Read the model definition and answer for the solid it produces. Units are mm, in the model's axes. Face numbers are marked on the shaded views. A direction names the side the tool comes from. Round coordinates to 2 decimals unless told otherwise and drop trailing zeros. Loops run counter-clockwise (first coordinate to the right, second up) from the corner with the lowest first, then second, coordinate; pieces in that order, holes last. Notation, with made-up numbers: M 16.5,-25.75 L 38.5,-25.75 A21 cw 38.5,1.25 Z; hole C -13,62.5 d4. An arc over 180 degrees is marked long. Write each question's results on one line, items separated by ' | '.
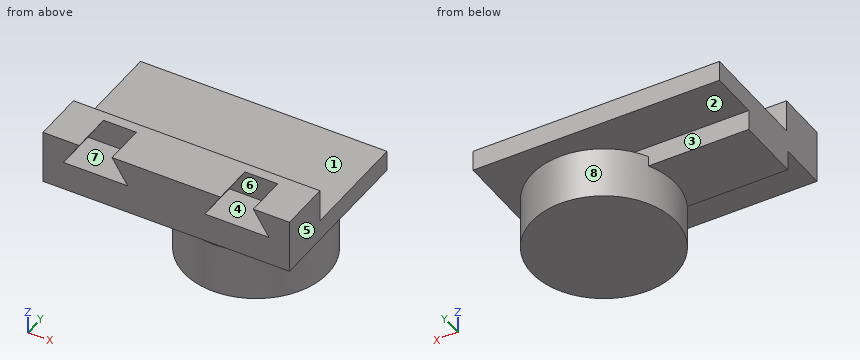
```python
from build123d import *

# Parameters (mm, degrees)
F0_W      = 38.1
F0_H      = 25.4
F1_DEPTH  = 3.175
F3_DEPTH  = 6.35
F4_W      = 38.1
F4_H      = 1.5875
F5_DEPTH  = 5.08
F6_R      = 11.1125
F7_DEPTH  = 9.525
F8_R      = 11.43
F8_R_2    = 7.62
F9_DEPTH  = 1.5875
F10_W     = 19.05
F10_H     = 10.16
F11_DEPTH = 3.175


with BuildPart() as f1:
    # F0 (on Top) → F1 (new body)
    with BuildSketch(Plane.XY):
        with Locations((-19.05, 12.7)):
            Rectangle(F0_W, F0_H)
    extrude(amount=F1_DEPTH)

    # F2 (on face) → F3 (join)
    with BuildSketch(Plane.XZ):
        Polygon((-38.1, 8.255), (-38.1, 3.175), (0, 3.175), (0, 8.255), (-5.588, 8.255), (-3.175, 4.445), (-13.081, 4.445), (-10.668, 8.255), (-27.432, 8.255), (-25.019, 4.445), (-34.925, 4.445), (-32.512, 8.255), align=None)
    extrude(amount=-F3_DEPTH)

    # F4 (on face) → F5 (join, through all)
    with BuildSketch(Plane.XY.offset(3.175)):
        with Locations((-19.05, 7.14375)):
            Rectangle(F4_W, F4_H)
    extrude(amount=F5_DEPTH)

    # F6 (on face) → F7 (join)
    with BuildSketch(Plane(origin=(0, 0, 0), x_dir=(1, 0, 0), z_dir=(0, 0, -1))):
        with Locations((-12.7, -12.7)):
            Circle(F6_R)
    extrude(amount=F7_DEPTH)

    # F8 (on face) → F9 (cut)
    with BuildSketch(Plane(origin=(0, 0, 0), x_dir=(1, 0, 0), z_dir=(0, 0, -1))):
        with Locations((-12.7, -12.7)):
            Circle(F8_R)
        with Locations((-12.7, -12.7)):
            Circle(F8_R_2, mode=Mode.SUBTRACT)
    extrude(amount=F9_DEPTH, mode=Mode.SUBTRACT)

    # F10 (on face) → F11 (join)
    with BuildSketch(Plane(origin=(0, 0, 0), x_dir=(1, 0, 0), z_dir=(0, 0, -1))):
        with Locations((-28.575, -12.7)):
            Rectangle(F10_W, F10_H)
    extrude(amount=F11_DEPTH)


solid = f1.part
```
1. Find section C-C, the plane y = 12.7. Give the vertices of the cut face in (x, z) (1 decimal), then the cut area to 3 significant figures.
Completed:
outline: M -38.1,-3.2 L -23.8,-3.2 L -23.8,-9.5 L -1.6,-9.5 L -1.6,-1.6 L -5.1,-1.6 L -5.1,0 L 0,0 L 0,3.2 L -38.1,3.2 Z | area: 372 mm2
2. Find section D-D, the plane z = -5.5. Give the vertices of the cut face in (x, y) (1 decimal), then the cut area to 3 significant figures.
Completed:
outline: C -12.7,12.7 d22.2 | area: 388 mm2
3. Find section A-A, the plane y = 22.5. Give the vertices of the cut face in (x, z) (1 decimal), then the cut area to 3 significant figures.
Completed:
outline: M -38.1,0 L 0,0 L 0,3.2 L -38.1,3.2 Z; M -17.9,-9.5 L -7.5,-9.5 L -7.5,-1.6 L -17.9,-1.6 Z | area: 204 mm2
4. Given P1, Ø6.5, axis at x = -16.5, y = 18, coming from the +Z side (3 decimals); P2, Ø1.9, axis at x = -9, z = 7, coming from the -Y side; P3, Ø1, axis at y = 17.5, z = -1, coming from the +X side, each flat-ended and moving along its own axis, determine where each tip first touches the part or whether it passes through.
Completed:
P1: stops at z = 3.175 | P2: stops at y = 6.35 | P3: stops at x = -6.41
5. Determine the mould class of the marked faces 5, 6, 7 and 8 for opening direction X: released by +X, released by -X, zero draft, split by the parting line, or undercut.
Completed:
face 5: released by +X | face 6: undercut | face 7: undercut | face 8: split by the parting line
6. Which of the six approach directions +Z, -Z, +X, -X, +Y, -Y give full straight-line access (tool end or side, diameter ignored) to the marked faces 1, 2, 3 and 4?
Completed:
face 1: +Z, +X, -X, +Y | face 2: none | face 3: -X, +Y | face 4: -Y
7. Find the intervals of material crossed by L1, parallel to Z at x = -12, y = 22.25 (1 decimal); L2, parallel to Z at x = -18, y = 11.5 (3 decimals); L3, parallel to Z at x = -33.5, y = 22.5 (3 decimals), in increasing order.
Completed:
L1: z = -9.5 to -1.6, 0 to 3.2 | L2: z = -9.525 to 3.175 | L3: z = 0 to 3.175
